Work out the finished part from the listing and answer in its coordinate system (mm). A direction names the side the tool comes from. Give positions to 0.01 mm unless a question says otherwise; leave off trailing zeros. Loops run counter-clockwise (first coordinate to the right, second up) from the corner with the lowest first, then second, coordinate; pieces in that order, holes last. Notation, with made-up numbers: (-19, -35.5) - (18, -35.5) arc R17 cw to (18, -8.5) - close; hole circle Ø4 at (18, 75.5). An arc over 180 degrees is marked (long way). One line per question, with ' | ' between items. Start each with the question number.
1. Each of these flat-tipped pins is pushed along its axis until it touches: pin 1 (2 mm diameter, centred on y = 2.5, z = -21.5, fed in from -X); pin 2 (3 mm diameter, centred on x = 23, z = -83.8, fed in from -Y); pin 3 (2.5 mm diameter, centred on x = 19, z = -55.5, fed in from +Y). Where does it stop, or does it pass through?
2. Which of the six approach directions +Z, -Z, +X, -X, +Y, -Y give full straight-line access (tool end or side, diameter ignored) to faces 1 (the face through (15, 2, -88.4)), 2 (the face through (40, 2, -44)), 3 (the face through (20, 2, -40.2)), 4 (the face through (22, 2.5, -4)), 5 (the face through (20, 2, -52))?
3. Section B-B (z = -57) is taken. Determine the outline of the cut face in (x, y), plus the area to 3 significant figures.
4. Section C-C (z = -83.8) is taken. Determine the outline of the cut face in (x, y).
5. Find the intervals of material crossed by line 1 (Z direction, x = 18.5, y = 0.9); line 2 (Z direction, x = 20.5, y = 3.55); line 3 (X direction, y = 3.45, z = -49), in increasing order.
6. Section A-A (y = 1.4) is taken. Determine the outline of the cut face in (x, z), plus the area to 3 significant figures.
7. For a pull along X with two mould halves and no side action, classify faces 6 (the face through (15, 2, 0)), 7 (the face through (22.3, 2.5, -47.8)), 8 (the face through (37.15, 2.03, -85.39)) as released by +X, released by -X, zero draft, split by the parting line, or undercut.
8. Section D-D (x = 35.5) is taken. Determine the outline of the cut face in (y, z), plus the area to 3 significant figures.
from build123d import *

# Parameters (mm, degrees)
SKETCH1_W           = 40
SKETCH1_H           = 88.4
BOSS_EXTRUDE1_DEPTH = 4
FILLET1_R           = 10
SKETCH3_R           = 1
CUT_EXTRUDE1_DEPTH  = 10
SKETCH5_R           = 1.6
CUT_EXTRUDE2_DEPTH  = 2.5
CUT_EXTRUDE3_START  = -2
SKETCH6_W           = 4.6
SKETCH6_H           = 20
CUT_EXTRUDE3_DEPTH  = 10
SKETCH8_W           = 4.6
SKETCH8_H           = 3.6
CUT_EXTRUDE7_DEPTH  = 11.5


with BuildPart() as part:
    # Sketch1 → Boss-Extrude1 (new body)
    with BuildSketch(Plane(origin=(0, 0, 0), x_dir=(1, 0, 0), z_dir=(0, 1, 0))):
        with Locations((20, 44.2)):
            Rectangle(SKETCH1_W, SKETCH1_H)
    extrude(amount=BOSS_EXTRUDE1_DEPTH)

    # Fillet1
    fillet1_edges = [part.edges().sort_by_distance(p)[0] for p in [
        (40, 2, -88.4),
        (40, 2, 0),
    ]]
    fillet(fillet1_edges, radius=FILLET1_R)

    # Sketch3 → Cut-Extrude1 (cut)
    with BuildSketch(Plane.XZ):
        with Locations(Location((23, -4.6, 0), (0, 0, 270))):
            Circle(SKETCH3_R)
        with Locations(Location((23, -83.8, 0), (0, 0, 270))):
            Circle(SKETCH3_R)
    extrude(amount=-CUT_EXTRUDE1_DEPTH, mode=Mode.SUBTRACT)

    # Sketch5 → Cut-Extrude2 (cut)
    with BuildSketch(Plane.XZ):
        with Locations(Location((23, -4.6, 0), (0, 0, 270))):
            Circle(SKETCH5_R)
        with Locations(Location((23, -83.8, 0), (0, 0, 270))):
            Circle(SKETCH5_R)
    extrude(amount=-CUT_EXTRUDE2_DEPTH, mode=Mode.SUBTRACT)

    # Sketch6 → Cut-Extrude3 (cut)
    with BuildSketch(Plane.XZ.offset(CUT_EXTRUDE3_START)):
        with Locations((20, -50.2)):
            Rectangle(SKETCH6_W, SKETCH6_H)
    extrude(amount=-CUT_EXTRUDE3_DEPTH, mode=Mode.SUBTRACT)

    # Sketch8 → Cut-Extrude7 (cut)
    with BuildSketch(Plane(origin=(0, 2, 0), x_dir=(1, 0, 0), z_dir=(0, 1, 0))):
        with Locations((20, 42)):
            Rectangle(SKETCH8_W, SKETCH8_H)
    extrude(amount=-CUT_EXTRUDE7_DEPTH, mode=Mode.SUBTRACT)


solid = part.part
Conclusion:
1) pin 1: x = 0 | pin 2: y = 2.5 | pin 3: y = 2
2) face 1: -Z, +X, -X, +Y, -Y | face 2: +Z, -Z, +X, +Y, -Y | face 3: +Y, -Y | face 4: -Y | face 5: +Y
3) outline: (0, 0) - (40, 0) - (40, 4) - (22.3, 4) - (22.3, 2) - (17.7, 2) - (17.7, 4) - (0, 4) - close | area: 151 mm²
4) outline: (0, 0) - (21.4, 0) - (21.4, 2.5) - (22, 2.5) - (22, 4) - (0, 4) - close; (24, 2.5) - (24.6, 2.5) - (24.6, 0) - (38.42, 0) - (38.42, 4) - (24, 4) - close
5) line 1: -88.4 to -43.8, -40.2 to 0 | line 2: -88.4 to -60.2, -40.2 to 0 | line 3: 0 to 17.7, 22.3 to 40
6) outline: (0, -88.4) - (30, -88.4) arc R10 ccw to (40, -78.4) - (40, -10) arc R10 ccw to (30, 0) - (0, 0) - close; hole (17.7, -43.8) - (22.3, -43.8) - (22.3, -40.2) - (17.7, -40.2) - close; hole circle Ø3.2 at (23, -83.8); hole circle Ø3.2 at (23, -4.6) | area: 3,460 mm²
7) face 6: zero draft | face 7: undercut | face 8: released by +X
8) outline: (0, -86.75) - (4, -86.75) - (4, -1.65) - (0, -1.65) - close | area: 340 mm²
